Design review of the part built by this model. Coordinates are the model's own, in mm. Give positions to 0.01 mm unless a question says otherwise; leave off trailing zeros. Loops run counter-clockwise (first coordinate to the right, second up) from the corner with the lowest first, then second, coordinate; pieces in that order, holes last. Notation, with made-up numbers: (48, 16.5) - (80, 16.5) arc R31 cw to (80, 43.5) - close; hole circle Ø11 at (-30, -37.5). An arc over 180 degrees is marked (long way). Put each result on its own line as item: value. Start each with the question number.
```python
from build123d import *

# Parameters (mm, degrees)
MODEL_R             = 1.397
MODEL_W             = 11.572
MODEL_H             = 3.17
MODEL_W_2           = 3.17
MODEL_H_2           = 29.8065
MODEL_W_3           = 43.464000078
BOSS_EXTRUDE1_DEPTH = 3.048
SKETCH2_R           = 3.810000039
SKETCH2_R_2         = 2
SKETCH2_R_3         = 3.809999961
BOSS_EXTRUDE2_DEPTH = 3.048
SKETCH3_R           = 2.49
CUT_EXTRUDE1_DEPTH  = 4.048


with BuildPart() as part:
    # Model → Boss-Extrude1 (new body)
    with BuildSketch(Plane.XY):
        with BuildLine():
            Line((26.3398, 0), (2.54, 0))
            ThreePointArc((2.54, 0), (0.743948776, 0.743948776), (0, 2.54))
            Line((0, 2.54), (0, 97.154990539))
            ThreePointArc((0, 97.154990539), (0.743948776, 98.951041763), (2.54, 99.694990539))
            Line((2.54, 99.694990539), (64.77, 99.694990539))
            ThreePointArc((64.77, 99.694990539), (66.566051224, 98.951041763), (67.31, 97.154990539))
            Line((67.31, 97.154990539), (67.31, 2.54))
            ThreePointArc((67.31, 2.54), (66.566051224, 0.743948776), (64.77, 0))
            Line((64.77, 0), (43.815, 0))
            Line((43.815, 0), (43.815, 11.0744))
            Line((43.815, 11.0744), (26.3398, 11.0744))
            Line((26.3398, 11.0744), (26.3398, 0))
        make_face()
        with Locations((9.144, 9.144)):
            Circle(MODEL_R, mode=Mode.SUBTRACT)
        with Locations((58.166, 9.144)):
            Circle(MODEL_R, mode=Mode.SUBTRACT)
        with Locations((9.144, 67.183)):
            Circle(MODEL_R, mode=Mode.SUBTRACT)
        with Locations((58.166, 67.183)):
            Circle(MODEL_R, mode=Mode.SUBTRACT)
        with Locations((52.771, 3.998)):
            Rectangle(MODEL_W, MODEL_H, mode=Mode.SUBTRACT)
        with Locations((63.312, 26.82625)):
            Rectangle(MODEL_W_2, MODEL_H_2, mode=Mode.SUBTRACT)
        with Locations((63.312, 69.31275)):
            Rectangle(MODEL_W_2, MODEL_H_2, mode=Mode.SUBTRACT)
        with Locations((33.654999961, 92.141)):
            Rectangle(MODEL_W_3, MODEL_H, mode=Mode.SUBTRACT)
        with Locations((3.997999922, 69.31275)):
            Rectangle(MODEL_W_2, MODEL_H_2, mode=Mode.SUBTRACT)
        with Locations((3.997999922, 26.82625)):
            Rectangle(MODEL_W_2, MODEL_H_2, mode=Mode.SUBTRACT)
        with Locations((14.538999922, 3.998)):
            Rectangle(MODEL_W, MODEL_H, mode=Mode.SUBTRACT)
    extrude(amount=BOSS_EXTRUDE1_DEPTH)

    # Sketch2 → Boss-Extrude2 (add)
    with BuildSketch(Plane.XY.offset(3.048)):
        with BuildLine():
            Line((-3.810000039, 74.929999922), (0, 74.929999922))
            Line((0, 74.929999922), (0, 78.739999961))
            ThreePointArc((0, 78.739999961), (-1.115923175, 76.045923097), (-3.810000039, 74.929999922))
        make_face()
        with Locations((-3.810000039, 78.739999961)):
            Circle(SKETCH2_R)
        with Locations((-3.810000039, 78.739999961)):
            Circle(SKETCH2_R_2, mode=Mode.SUBTRACT)
        with BuildLine():
            ThreePointArc((-3.810000039, 82.55), (-1.115923175, 81.434076825), (0, 78.739999961))
            Line((0, 78.739999961), (0, 82.55))
            Line((0, 82.55), (-3.810000039, 82.55))
        make_face()
        with BuildLine():
            Line((67.31, 78.739999961), (67.31, 74.929999922))
            Line((67.31, 74.929999922), (71.119999961, 74.929999922))
            ThreePointArc((71.119999961, 74.929999922), (68.425923097, 76.045923097), (67.309999922, 78.739999961))
        make_face()
        with BuildLine():
            Line((67.31, 82.55), (67.31, 78.739999961))
            ThreePointArc((67.309999922, 78.739999961), (68.425923097, 81.434076825), (71.119999961, 82.55))
            Line((71.119999961, 82.55), (67.31, 82.55))
        make_face()
        with BuildLine():
            ThreePointArc((67.31, 2.54), (66.566051224, 0.743948776), (64.77, 0))
            Line((64.77, 0), (71.119999961, 0))
            ThreePointArc((71.119999961, 0), (68.425923152, 1.115923152), (67.31, 3.809999961))
            Line((67.31, 3.809999961), (67.31, 2.54))
        make_face()
        with Locations((71.119999961, 3.809999961)):
            Circle(SKETCH2_R_3)
        with Locations((71.119999961, 3.809999961)):
            Circle(SKETCH2_R_2, mode=Mode.SUBTRACT)
        with BuildLine():
            Line((67.31, 7.619999922), (67.31, 3.809999961))
            ThreePointArc((67.31, 3.809999961), (68.425923152, 6.50407677), (71.119999961, 7.619999922))
            Line((71.119999961, 7.619999922), (67.31, 7.619999922))
        make_face()
        with BuildLine():
            ThreePointArc((-7.8e-08, 3.809999961), (-1.11592323, 1.115923152), (-3.810000039, 0))
            Line((-3.810000039, 0), (2.54, 0))
            ThreePointArc((2.54, 0), (0.743948776, 0.743948776), (0, 2.54))
            Line((0, 2.54), (0, 3.809999961))
        make_face()
        with Locations((-3.810000039, 3.809999961)):
            Circle(SKETCH2_R_3)
        with Locations((-3.810000039, 3.809999961)):
            Circle(SKETCH2_R_2, mode=Mode.SUBTRACT)
        with BuildLine():
            Line((0, 7.619999922), (-3.810000039, 7.619999922))
            ThreePointArc((-3.810000039, 7.619999922), (-1.11592323, 6.50407677), (-7.8e-08, 3.809999961))
            Line((0, 3.809999961), (0, 7.619999922))
        make_face()
        with Locations((71.119999961, 78.739999961)):
            Circle(SKETCH2_R)
        with Locations((71.119999961, 78.739999961)):
            Circle(SKETCH2_R_2, mode=Mode.SUBTRACT)
    extrude(amount=-BOSS_EXTRUDE2_DEPTH)

    # Sketch3 → Cut-Extrude1 (cut, through all)
    with BuildSketch(Plane(origin=(0, 0, 0), x_dir=(-1, 0, 0), z_dir=(0, 0, -1))):
        with Locations((-29.649999961, 60.0845)):
            Circle(SKETCH3_R)
        with Locations((-37.659999961, 60.0845)):
            Circle(SKETCH3_R)
        with Locations((-37.659999961, 52.0745)):
            Circle(SKETCH3_R)
        with Locations((-29.649999961, 52.0745)):
            Circle(SKETCH3_R)
        with Locations((-29.649999961, 44.0645)):
            Circle(SKETCH3_R)
        with Locations((-37.659999961, 44.0645)):
            Circle(SKETCH3_R)
        with Locations((-29.649999961, 36.0545)):
            Circle(SKETCH3_R)
        with Locations((-37.659999961, 36.0545)):
            Circle(SKETCH3_R)
    extrude(amount=-CUT_EXTRUDE1_DEPTH, mode=Mode.SUBTRACT)


solid = part.part
```
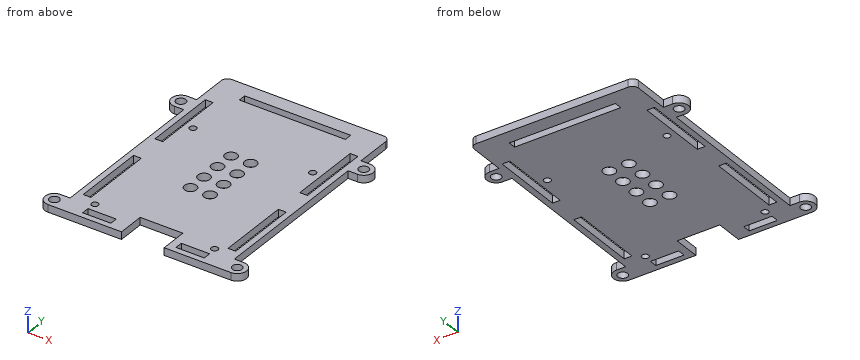
Item 1: Consider section B-B (x = 37.66). State the section outline as (y, z) points (1 decimal).
Item 2: Consider section A-A (y = 3.81). State the section outline as (x, z) points (3 decimals).
Item 3: Consider section C-C (y = 72.5). State the section outline as (x, z) points.
Item 4: Consider section D-D (x = 63). State the section outline as (y, z) points (1 decimal).
Item 5: For L1, parallel to X at y = 74, z = 1.65; L2, parallel to Y at x = 37.66, z = 1.5 (1 decimal); L3, parallel to X at y = 3.81, z = 1.3 (3 decimals), list the stretches that pass through material, from the lowest coordinate up. Write a range as from..to.
Item 6: For P1, Ø1.5, axis at x = 69.5, z = 1.5, coming from the +Y side; P2, Ø0.9, axis at y = 65, z = 2, coming from the -X side; P3, Ø1.5, axis at y = 86.5, z = 1, coming from the +X side, all flat-tipped, find the tip position at first contact; note any pin that passes through.
Geometry says:
1. outline: (11.1, 0) - (33.6, 0) - (33.6, 3) - (11.1, 3) - close; (38.5, 0) - (41.6, 0) - (41.6, 3) - (38.5, 3) - close; (46.6, 0) - (49.6, 0) - (49.6, 3) - (46.6, 3) - close; (54.6, 0) - (57.6, 0) - (57.6, 3) - (54.6, 3) - close; (62.6, 0) - (90.6, 0) - (90.6, 3) - (62.6, 3) - close; (93.7, 0) - (99.7, 0) - (99.7, 3) - (93.7, 3) - close
2. outline: (-7.62, 0) - (-5.81, 0) - (-5.81, 3.048) - (-7.62, 3.048) - close; (-1.81, 0) - (8.753, 0) - (8.753, 3.048) - (-1.81, 3.048) - close; (20.325, 0) - (26.34, 0) - (26.34, 3.048) - (20.325, 3.048) - close; (43.815, 0) - (46.985, 0) - (46.985, 3.048) - (43.815, 3.048) - close; (58.557, 0) - (69.12, 0) - (69.12, 3.048) - (58.557, 3.048) - close; (73.12, 0) - (74.93, 0) - (74.93, 3.048) - (73.12, 3.048) - close
3. outline: (0, 0) - (2.41, 0) - (2.41, 3.05) - (0, 3.05) - close; (5.58, 0) - (61.73, 0) - (61.73, 3.05) - (5.58, 3.05) - close; (64.9, 0) - (67.31, 0) - (67.31, 3.05) - (64.9, 3.05) - close
4. outline: (0, 0) - (11.9, 0) - (11.9, 3) - (0, 3) - close; (41.7, 0) - (54.4, 0) - (54.4, 3) - (41.7, 3) - close; (84.2, 0) - (99.7, 0) - (99.7, 3) - (84.2, 3) - close
5. L1: x = 0..2.41, 5.58..61.73, 64.9..67.31
5. L2: y = 11.1..33.6, 38.5..41.6, 46.6..49.6, 54.6..57.6, 62.6..90.6, 93.7..99.7
5. L3: x = -7.62..-5.81, -1.81..8.753, 20.325..26.34, 43.815..46.985, 58.557..69.12, 73.12..74.93
6. P1: stops at y = 82.55
6. P2: stops at x = 0
6. P3: stops at x = 67.31
